Can you work these out from the drawing? Everything is in mm from the part's minimum corner. Give positions to 0.01 mm unless a question says otherwise; leave off trailing zeros. Order: outer loops, then holes, each group sorted by start corner. A loop starts at its lowest first (then second) coordinate and runs counter-clockwise, first axis right, second up. Notation, with made-up numbers: M 40.5,41.25 L 92.5,41.25 A23 cw 92.5,53.25 Z; hole C 67,25.25 d9. An arc over 180 degrees is marked long. Use a Markdown table: item, result. Add a question column.
Item 1: Suppose I cut it at B-B on z = 1.3. Count the separate pieces of the cut face and the enclosed holes in it, plus the area to 3 significant figures.
Item 2: If I drill on L1, parallel to Y at x = 63.5, z = 1.6; L2, parallel to X at y = 13.5, z = 1.4; L3, parallel to X at y = 15, z = 2.9, over which ranges is the centre line in solid material (lowest first)? Write a range as from..to.
Item 3: Suppose I cut it at A-A on x = 12.7. Write out the boundary of the cut face in (y, z), plus the area to 3 significant figures.
Item 4: Suppose I cut it at C-C on y = 2. Write out the boundary of the cut face in (x, z).
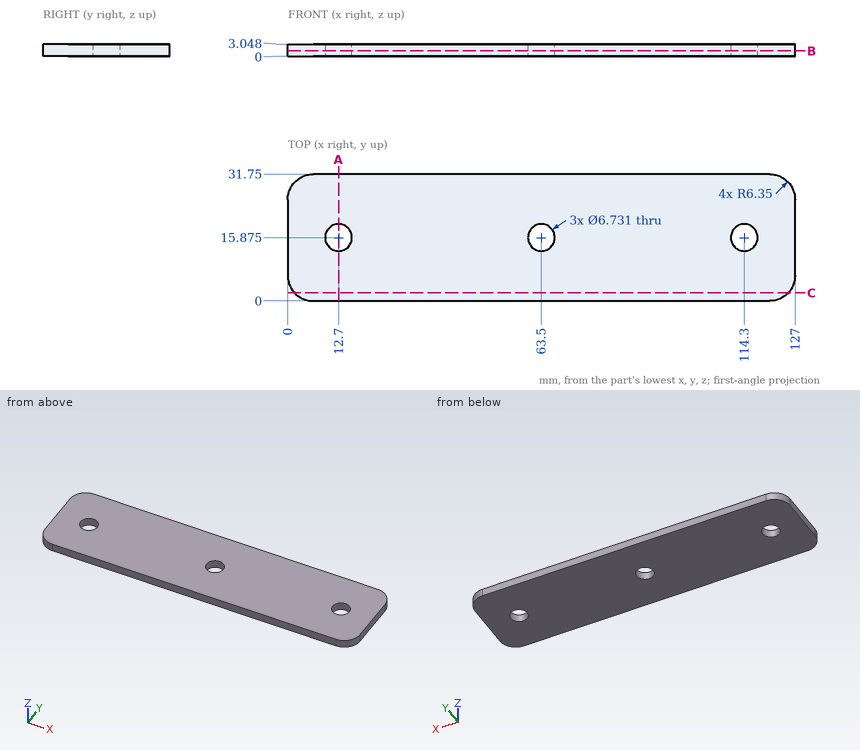
Findings below:
| question | item | result |
|---|---|---|
| 1 | separate pieces | 1 |
| 1 | enclosed holes | 3 |
| 1 | area | 3,890 mm^2 |
| 2 | L1 | y = 0..12.51, 19.24..31.75 |
| 2 | L2 | x = 0..10.32, 15.08..61.12, 65.88..111.92, 116.68..127 |
| 2 | L3 | x = 0..9.45, 15.95..60.25, 66.75..111.05, 117.55..127 |
| 3 | outline | M 0,0 L 12.51,0 L 12.51,3.05 L 0,3.05 Z; M 19.24,0 L 31.75,0 L 31.75,3.05 L 19.24,3.05 Z |
| 3 | area | 76.3 mm^2 |
| 4 | outline | M 1.72,0 L 125.28,0 L 125.28,3.05 L 1.72,3.05 Z |
